Build history of the part. All positions in model axes, mm. Face numbers are marked on the shaded views. A direction names the side the tool comes from. Round coordinates to 2 decimals unless told otherwise and drop trailing zeros. Loops run counter-clockwise (first coordinate to the right, second up) from the corner with the lowest first, then second, coordinate; pieces in that order, holes last. Notation, with made-up numbers: (72, 21) - (128, 21) arc R10 cw to (128, 35) - close; hole circle Ø10 at (50, 71.25). An arc over 180 degrees is marked (long way). Use one line per item in the form item = value. Start each with the question number.
Q1. Saw through at D-D (z = 1.5). Give the cut face in (x, y), then the cut area to 3 significant figures.
Q2. Saw through at C-C (y = 0). Give the cut face in (x, z).
Q3. Saw through at B-B (z = 3.5). Give the cut face in (x, y).
Q4. 3-axis set-ups, long thin cutter, end or side, ignore diameter. For the marked faces 5, 6, 7 and 8: which of +Z, -Z, +X, -X, +Y, -Y reach the whole face in a straight line?
Q5. Pin check, flat tips, straight feed: pin 1 (0.6 mm diameter, centred on y = -12.5, z = 2, fed in from +X); pin 2 (0.8 mm diameter, centred on x = 1.5, z = 6, fed in from +Y); pin 3 (4 mm diameter, centred on x = -0.5, y = -18.5, fed in from +Z); pin 4 (2.5 mm diameter, centred on x = 0, y = 0, fed in from +Z). Stop position of each tip, or through.
Q6. Saw through at A-A (x = 0). Give the cut face in (y, z).
Q7. Drill centre lines: line 1 (Y direction, x = -4.98, z = 3.5); line 2 (Y direction, x = -0.25, z = 2.75); line 3 (Z direction, x = -0.75, y = -24.5). Where is each one in solid material? Low to high.
Q8. Mould opens along X. For the marked faces 1, 2, 3 and 4 say: released by +X, released by -X, zero draft, split by the parting line, or undercut.
```python
from build123d import *

# Parameters (mm, degrees)
SKETCH1_R       = 2.15
SKETCH1_R_2     = 1.5
EXTRUDE1_DEPTH  = 3
SKETCH2_R       = 6
SKETCH2_R_2     = 2.15
EXTRUDE2_DEPTH  = 6
EXTRUDE3_DEPTH  = 3
SKETCH4_R       = 1.5
EXTRUDE4_DEPTH  = 4.5
FILLET5_R       = 1
CHAMFER1_SIZE   = 6
CHAMFER1_SIZE_2 = 1.949518177


with BuildPart() as part:
    # Sketch1 → Extrude1 (new body)
    with BuildSketch(Plane.XY):
        with BuildLine():
            Line((-7.48, -27), (7.48, -27))
            ThreePointArc((7.48, -27), (8.894213562, -26.414213562), (9.48, -25))
            Line((9.48, -25), (9.48, -23.15))
            Line((9.48, -23.15), (5.935760988, 0.875637761))
            ThreePointArc((5.935760988, 0.875637761), (0, 6), (-5.935760988, 0.875637761))
            Line((-5.935760988, 0.875637761), (-9.48, -23.15))
            Line((-9.48, -23.15), (-9.48, -25))
            ThreePointArc((-9.48, -25), (-8.894213562, -26.414213562), (-7.48, -27))
        make_face()
        Circle(SKETCH1_R, mode=Mode.SUBTRACT)
        with Locations((-4.98, -23.2)):
            Circle(SKETCH1_R_2, mode=Mode.SUBTRACT)
        with Locations((4.98, -23.2)):
            Circle(SKETCH1_R_2, mode=Mode.SUBTRACT)
    extrude(amount=EXTRUDE1_DEPTH)

    # Sketch2 → Extrude2 (add)
    with BuildSketch(Plane.XY.offset(3)):
        with Locations(Location((0, 0, 0), (0, 0, 171.608305322))):
            Circle(SKETCH2_R)
        Circle(SKETCH2_R_2, mode=Mode.SUBTRACT)
    extrude(amount=EXTRUDE2_DEPTH)

    # Sketch3 → Extrude3 (cut)
    with BuildSketch(Plane.XY.offset(3)):
        with BuildLine():
            Line((-4, -10.5), (4, -10.5))
            ThreePointArc((4, -10.5), (4.707106781, -10.792893219), (5, -11.5))
            Line((5, -11.5), (5, -13.5))
            ThreePointArc((5, -13.5), (4.707106781, -14.207106781), (4, -14.5))
            Line((4, -14.5), (-4, -14.5))
            ThreePointArc((-4, -14.5), (-4.707106781, -14.207106781), (-5, -13.5))
            Line((-5, -13.5), (-5, -11.5))
            ThreePointArc((-5, -11.5), (-4.707106781, -10.792893219), (-4, -10.5))
        make_face()
    extrude(amount=-EXTRUDE3_DEPTH, mode=Mode.SUBTRACT)

    # Sketch4 → Extrude4 (add)
    with BuildSketch(Plane.XY.offset(3)):
        with BuildLine():
            Line((-7.48, -27), (7.48, -27))
            ThreePointArc((7.48, -27), (8.894213562, -26.414213562), (9.48, -25))
            Line((9.48, -25), (9.48, -23.15))
            Line((9.48, -23.15), (8.823540273, -18.7))
            Line((8.823540273, -18.7), (-8.823540273, -18.7))
            Line((-8.823540273, -18.7), (-9.48, -23.15))
            Line((-9.48, -23.15), (-9.48, -25))
            ThreePointArc((-9.48, -25), (-8.894213562, -26.414213562), (-7.48, -27))
        make_face()
        with Locations((-4.98, -23.2)):
            Circle(SKETCH4_R, mode=Mode.SUBTRACT)
        with Locations((4.98, -23.2)):
            Circle(SKETCH4_R, mode=Mode.SUBTRACT)
    extrude(amount=EXTRUDE4_DEPTH)

    # Fillet5
    # the kernel refuses this fillet: 1 mm, written as the material it adds along each edge
    with BuildSketch(Plane(origin=(14.823540273, -18.7, 3), x_dir=(0, 0, 1), z_dir=(-1, 0, 0))) as fillet5_piece_1_section:
        with BuildLine():
            CenterArc((FILLET5_R, FILLET5_R), FILLET5_R, 180, 90)
            Line((0, FILLET5_R), (-FILLET5_R * 0.02, FILLET5_R))
            Line((-FILLET5_R * 0.02, FILLET5_R), (-FILLET5_R * 0.02, -FILLET5_R * 0.02))
            Line((-FILLET5_R * 0.02, -FILLET5_R * 0.02), (FILLET5_R, -FILLET5_R * 0.02))
            Line((FILLET5_R, -FILLET5_R * 0.02), (FILLET5_R, 0))
        make_face()
    fillet5_piece_1 = extrude(amount=29.647080546, mode=Mode.PRIVATE)
    fillet5_piece_1 = split(fillet5_piece_1, bisect_by=Plane(origin=(-8.603039543, -17.20527274, 3.226855902), z_dir=(0.9892934980650984, -0.1459396268534398, 0)), keep=Keep.TOP, mode=Mode.PRIVATE)
    fillet5_piece_1 = split(fillet5_piece_1, bisect_by=Plane(origin=(8.603039543, -17.20527274, 3.226855902), z_dir=(-0.9892934980650984, -0.14593962685343984, 0)), keep=Keep.TOP, mode=Mode.PRIVATE)
    add(fillet5_piece_1)
    # the kernel refuses this fillet: 1 mm, written as the material it takes off along each edge
    with BuildSketch(Plane(origin=(-9.48, -17.15, 7.5), x_dir=(0, 0, -1), z_dir=(0, -1, 0))) as fillet5_2_piece_1:
        with BuildLine():
            CenterArc((FILLET5_R, FILLET5_R), FILLET5_R, 180, 90)
            Line((0, FILLET5_R), (-FILLET5_R * 0.02, FILLET5_R))
            Line((-FILLET5_R * 0.02, FILLET5_R), (-FILLET5_R * 0.02, -FILLET5_R * 0.02))
            Line((-FILLET5_R * 0.02, -FILLET5_R * 0.02), (FILLET5_R, -FILLET5_R * 0.02))
            Line((FILLET5_R, -FILLET5_R * 0.02), (FILLET5_R, 0))
        make_face()
    extrude(amount=7.85, mode=Mode.SUBTRACT)
    with BuildSketch(Plane(origin=(9.48, -25, 7.5), x_dir=(-1, 0, 0), z_dir=(0, 1, 0))) as fillet5_2_piece_2:
        with BuildLine():
            CenterArc((FILLET5_R, -FILLET5_R), FILLET5_R, 90, 90)
            Line((0, -FILLET5_R), (-FILLET5_R * 0.02, -FILLET5_R))
            Line((-FILLET5_R * 0.02, -FILLET5_R), (-FILLET5_R * 0.02, FILLET5_R * 0.02))
            Line((-FILLET5_R * 0.02, FILLET5_R * 0.02), (FILLET5_R, FILLET5_R * 0.02))
            Line((FILLET5_R, FILLET5_R * 0.02), (FILLET5_R, 0))
        make_face()
    extrude(amount=7.85, mode=Mode.SUBTRACT)
    with BuildSketch(Plane(origin=(-7.48, -27, 7.5), x_dir=(0, 1, 0), z_dir=(1, 0, 0))) as fillet5_2_piece_3:
        with BuildLine():
            CenterArc((FILLET5_R, -FILLET5_R), FILLET5_R, 90, 90)
            Line((0, -FILLET5_R), (-FILLET5_R * 0.02, -FILLET5_R))
            Line((-FILLET5_R * 0.02, -FILLET5_R), (-FILLET5_R * 0.02, FILLET5_R * 0.02))
            Line((-FILLET5_R * 0.02, FILLET5_R * 0.02), (FILLET5_R, FILLET5_R * 0.02))
            Line((FILLET5_R, FILLET5_R * 0.02), (FILLET5_R, 0))
        make_face()
    extrude(amount=14.96, mode=Mode.SUBTRACT)
    with BuildSketch(Plane(origin=(14.823540273, -18.7, 7.5), x_dir=(0, -1, 0), z_dir=(-1, 0, 0))) as fillet5_2_piece_4:
        with BuildLine():
            CenterArc((FILLET5_R, -FILLET5_R), FILLET5_R, 90, 90)
            Line((0, -FILLET5_R), (-FILLET5_R * 0.02, -FILLET5_R))
            Line((-FILLET5_R * 0.02, -FILLET5_R), (-FILLET5_R * 0.02, FILLET5_R * 0.02))
            Line((-FILLET5_R * 0.02, FILLET5_R * 0.02), (FILLET5_R, FILLET5_R * 0.02))
            Line((FILLET5_R, FILLET5_R * 0.02), (FILLET5_R, 0))
        make_face()
    extrude(amount=29.647080546, mode=Mode.SUBTRACT)
    with BuildSketch(Plane(origin=(-7.48, -25, 7.5), x_dir=(-1, 0, 0), z_dir=(0, 1, 0))) as fillet5_2_piece_5:
        with BuildLine():
            CenterArc((2 - FILLET5_R, -FILLET5_R), FILLET5_R, 0, 90)
            Line((2, -FILLET5_R), (2 + FILLET5_R * 0.02, -FILLET5_R))
            Line((2 + FILLET5_R * 0.02, -FILLET5_R), (2 + FILLET5_R * 0.02, FILLET5_R * 0.02))
            Line((2 + FILLET5_R * 0.02, FILLET5_R * 0.02), (2 - FILLET5_R, FILLET5_R * 0.02))
            Line((2 - FILLET5_R, FILLET5_R * 0.02), (2 - FILLET5_R, 0))
        make_face()
    revolve(axis=Axis((-7.48, -25, 7.5), (0, 0, 1)), revolution_arc=90, mode=Mode.SUBTRACT)
    with BuildSketch(Plane(origin=(7.48, -25, 7.5), x_dir=(0, -1, 0), z_dir=(-1, 0, 0))) as fillet5_2_piece_6:
        with BuildLine():
            CenterArc((2 - FILLET5_R, -FILLET5_R), FILLET5_R, 0, 90)
            Line((2, -FILLET5_R), (2 + FILLET5_R * 0.02, -FILLET5_R))
            Line((2 + FILLET5_R * 0.02, -FILLET5_R), (2 + FILLET5_R * 0.02, FILLET5_R * 0.02))
            Line((2 + FILLET5_R * 0.02, FILLET5_R * 0.02), (2 - FILLET5_R, FILLET5_R * 0.02))
            Line((2 - FILLET5_R, FILLET5_R * 0.02), (2 - FILLET5_R, 0))
        make_face()
    revolve(axis=Axis((7.48, -25, 7.5), (0, 0, 1)), revolution_arc=90, mode=Mode.SUBTRACT)

    # Chamfer1
    # the kernel refuses this chamfer: 6, 1.949518177 mm, written as the material it takes off along each edge
    with BuildSketch(Plane(origin=(0, 0, 9), x_dir=(-0.9892934980663286, 0.14593962684510065, 0), z_dir=(0.14593962684510065, 0.9892934980663286, 0))) as chamfer1_piece_1_section:
        Polygon((6, -CHAMFER1_SIZE), (6 - CHAMFER1_SIZE_2, 0), (6, 0), align=None)
    chamfer1_piece_1 = revolve(axis=Axis((0, 0, 9), (0, 0, 1)), mode=Mode.PRIVATE)
    chamfer1_piece_1 = split(chamfer1_piece_1, bisect_by=Plane(origin=(4.992893688, -0.736546882, 3), z_dir=(0, 0, 1)), keep=Keep.TOP, mode=Mode.PRIVATE)
    add(chamfer1_piece_1, mode=Mode.SUBTRACT)


solid = part.part
```
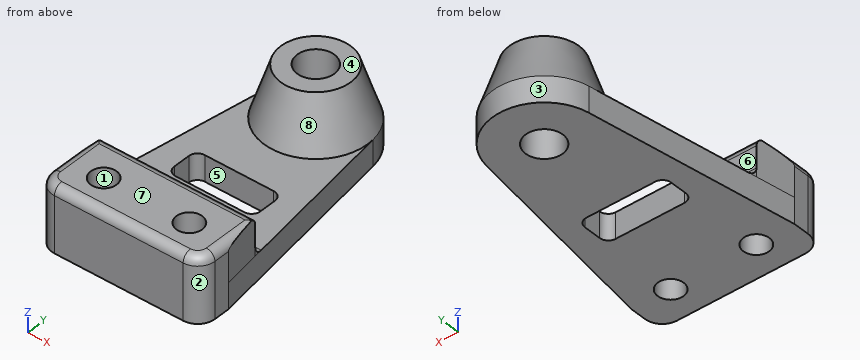
Report:
q1.outline = (-9.48, -25) arc R2 ccw to (-7.48, -27) - (7.48, -27) arc R2 ccw to (9.48, -25) - (9.48, -23.15) - (5.94, 0.88) arc R6 ccw to (-5.94, 0.88) - (-9.48, -23.15) - close; hole circle Ø3 at (-4.98, -23.2); hole (-5, -13.5) arc R1 ccw to (-4, -14.5) - (4, -14.5) arc R1 ccw to (5, -13.5) - (5, -11.5) arc R1 ccw to (4, -10.5) - (-4, -10.5) arc R1 ccw to (-5, -11.5) - close; hole circle Ø4.3 at (0, 0); hole circle Ø3 at (4.98, -23.2)
q1.area = 420 mm²
q2.outline = (-6.06, 0) - (-2.15, 0) - (-2.15, 9) - (-4.05, 9) - (-6, 3) - (-6.06, 3) - close; (2.15, 0) - (6.06, 0) - (6.06, 3) - (6, 3) - (4.05, 9) - (2.15, 9) - close
q3.outline = (-9.48, -25) arc R2 ccw to (-7.48, -27) - (7.48, -27) arc R2 ccw to (9.48, -25) - (9.48, -23.15) - (8.8, -18.57) - (-8.8, -18.57) - (-9.48, -23.15) - close; circle Ø11.68 at (0, 0); hole circle Ø3 at (-4.98, -23.2); hole circle Ø4.3 at (0, 0); hole circle Ø3 at (4.98, -23.2)
q4.face_5 = +Z, -Z
q4.face_6 = +Z, +X, -X
q4.face_7 = +Z, +X, -X, -Y
q4.face_8 = +Z
q5.pin_1 = 7.95
q5.pin_2 = 4.97
q5.pin_3 = 7.5
q5.pin_4 = through
q6.outline = (-27, 0) - (-14.5, 0) - (-14.5, 3) - (-17.7, 3) arc R1 cw to (-18.7, 4) - (-18.7, 6.5) arc R1 ccw to (-19.7, 7.5) - (-26, 7.5) arc R1 ccw to (-27, 6.5) - close; (-10.5, 0) - (-2.15, 0) - (-2.15, 9) - (-4.05, 9) - (-6, 3) - (-10.5, 3) - close; (2.15, 0) - (6, 0) - (6, 3) - (4.05, 9) - (2.15, 9) - close
q7.line_1 = -27 to -24.7, -21.7 to -18.57, -3.05 to 3.05
q7.line_2 = -27 to -14.5, -10.5 to -2.14, 2.14 to 5.99
q7.line_3 = 0 to 7.5
q8.face_1 = undercut
q8.face_2 = released by +X
q8.face_3 = split by the parting line
q8.face_4 = zero draft
